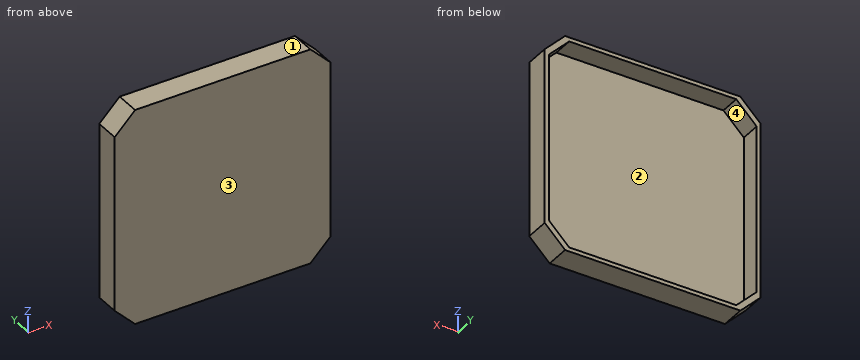
```python
from build123d import *

# Parameters (mm, degrees)
SKETCH1_W           = 106
SKETCH1_H           = 106
BOSS_EXTRUDE1_DEPTH = 2
SKETCH2_W           = 106
SKETCH2_H           = 106
SKETCH2_W_2         = 102
SKETCH2_H_2         = 102
BOSS_EXTRUDE2_DEPTH = 10
CHAMFER1_SIZE       = 10


with BuildPart() as part:
    # Sketch1 → Boss-Extrude1 (new body)
    with BuildSketch(Plane(origin=(0, 0, 0), x_dir=(1, 0, 0), z_dir=(0, 1, 0))):
        Rectangle(SKETCH1_W, SKETCH1_H)
    extrude(amount=BOSS_EXTRUDE1_DEPTH)

    # Sketch2 → Boss-Extrude2 (add)
    with BuildSketch(Plane(origin=(0, 2, 0), x_dir=(1, 0, 0), z_dir=(0, 1, 0))):
        Rectangle(SKETCH2_W, SKETCH2_H)
        Rectangle(SKETCH2_W_2, SKETCH2_H_2, mode=Mode.SUBTRACT)
    extrude(amount=BOSS_EXTRUDE2_DEPTH)

    # Chamfer1
    chamfer1_edges = [part.edges().sort_by_distance(p)[0] for p in [
        (-51, 7, -51),
        (-51, 7, 51),
        (51, 7, 51),
        (51, 7, -51),
        (-53, 6, -53),
        (53, 6, -53),
        (53, 6, 53),
        (-53, 6, 53),
    ]]
    chamfer(chamfer1_edges, length=CHAMFER1_SIZE)


solid = part.part
```
Model file for the job. Use its own axes, mm. Face numbers are marked on the shaded views. Give positions to 0.01 mm unless a question says otherwise; leave off trailing zeros. Order: outer loops, then holes, each group sorted by start corner. A loop starts at its lowest first (then second) coordinate and runs counter-clockwise, first axis right, second up.
1) Mould opens along Z. For the marked faces 1, 2, 3 and 4 say: +Z half, -Z half, draft (parallel to the pull), parting line (faces both ways), or undercut.
2) Saw through at B-B, the plane z = -46.5. Write the cut outline in (x, y), then the cut area to 3 significant figures.
3) Saw through at C-C, the plane x = 8. Write the cut outline in (y, z).
4) Wall check: probe 1 along Z at (x, y) = (-35.5, 8); probe 2 along Y at (x, z) = (18.5, -6). Give the ranges that are in metal, low to high.
5) Saw through at A-A, the plane y = 9.25. Write the cut outline in (x, z).
6) Pin check, flat tip, straight feed: pin 1 (2 mm diameter, centred on x = 36, z = -41.5, fed in from +Y). Stop position of the tip, or through.
Computed:
1. face 1: +Z half
1. face 2: undercut
1. face 3: draft
1. face 4: undercut
2. outline: (-49.5, 0) - (49.5, 0) - (49.5, 12) - (45.5, 12) - (45.5, 2) - (-45.5, 2) - (-45.5, 12) - (-49.5, 12) - close
2. area: 278 mm2
3. outline: (0, -53) - (12, -53) - (12, -51) - (2, -51) - (2, 51) - (12, 51) - (12, 53) - (0, 53) - close
4. probe 1: z = -53 to -51, 51 to 53
4. probe 2: y = 0 to 2
5. outline: (-53, -43) - (-43, -53) - (43, -53) - (53, -43) - (53, 43) - (43, 53) - (-43, 53) - (-53, 43) - close; hole (-51, -41) - (-41, -51) - (41, -51) - (51, -41) - (51, 41) - (41, 51) - (-41, 51) - (-51, 41) - close
6. pin 1: stops at y = 2
